from build123d import *

# Parameters (mm, degrees)
F1_DEPTH = 25


with BuildPart() as f1:
    # F0 (on Front) → F1 (new body)
    with BuildSketch(Plane.XZ):
        Polygon((42.157266, 36.458336), (0, 36.458336), (0, 32.877419), (39.633732, 32.877419), (39.633732, 12.629625), (35.397731, 12.629625), (35.397731, 8.376406), (39.750192, 8.376406), (39.750192, 6.429029), (39.750192, 6.314471), (49.760994, 6.314471), (49.760994, 8.376406), (49.683991, 10.766225), (42.157266, 10.766225), (42.157266, 12.629625), (42.157266, 14.715909), align=None)
    extrude(amount=F1_DEPTH)

    # F0 (on Front) → F2 (revolve)
    with BuildSketch(Plane.XZ):
        Polygon((42.157266, 36.458336), (0, 36.458336), (0, 32.877419), (39.633732, 32.877419), (39.633732, 12.629625), (35.397731, 12.629625), (35.397731, 8.376406), (39.750192, 8.376406), (39.750192, 6.429029), (39.750192, 6.314471), (49.760994, 6.314471), (49.760994, 8.376406), (49.683991, 10.766225), (42.157266, 10.766225), (42.157266, 12.629625), (42.157266, 14.715909), align=None)
    revolve(axis=Axis((0, 0, 20.221634), (0, 0, -1)))


solid = f1.part
Input: part model. Units: mm. Frame: model coordinates. A direction names the side the tool comes from. Round coordinates to 2 decimals unless told otherwise and drop trailing zeros. Loops run counter-clockwise (first coordinate to the right, second up) from the corner with the lowest first, then second, coordinate; pieces in that order, holes last. Notation, with made-up numbers: (0, 75) -> (23, 75) arc R4 ccw to (23, 80) -> close; hole circle Ø9 at (16.25, 74.25). An arc over 180 degrees is marked (long way). Answer as a JSON object with one key per item and string values. Group by question number.
1) Reachability of faces 5 (the flat face through (38, -22, 32.877)), 6 (the cylindrical face through (-31.54, 24.19, 7.33)), 7 (the flat face through (40, -25, 24)), 8 (the flat face through (1, -1, 32.877)) from +Z, -Z, +X, -X, +Y, -Y: full face, straight path, thin tool, end or side. Return the list, or none.
2) Pin query (flat end, axial travel): pin 1 (24 mm diameter, centred on x = -12.5, y = -19.5, fed in from -Z); pin 2 (8.5 mm diameter, centred on y = -18.5, z = 19, fed in from -X); pin 3 (4 mm diameter, centred on y = 1.5, z = 28, fed in from +X); pin 4 (1 mm diameter, centred on x = -25, y = 30.5, fed in from -Z). Return the tip coordinate at first contact, or that it passes through.
3) Ray query, L1, parallel to Y at x = 0, z = 7.9; L2, parallel to Y at x = 0, z = 11. Return the intervals inside material, ascending.
4) Draft query along Z for faces 1 (the conical face through (-48.467, 10.985, 10.385)), 2 (the cylindrical face through (33.763, -10.633, 10.473)), 3 (the flat face through (-14.9, -32.5, 12.63)), 4 (the flat face through (36, 3, 8.376)). Return one class per face: +Z half, -Z half, draft (parallel to the pull), parting line (faces both ways), or undercut.
5) Section query B-B on z = 19.5. Output: boundary loops of the cut face in (x, y).
6) Section query A-A on x = 0. Output: boundary loops of the cut face in (y, z), plus the area to 3 significant figures.
Reply:
{
 "1": {"face 5": "-Y", "face 6": "-Z", "face 7": "+Z, +X, -Y", "face 8": "none"},
 "2": {"pin 1": "stops at z = 32.88", "pin 2": "stops at x = -39.68", "pin 3": "stops at x = 42.16", "pin 4": "stops at z = 6.31"},
 "3": {"L1": "y = -49.76 to -39.75, 39.75 to 49.76", "L2": "y = -42.16 to -35.4, 35.4 to 42.16"},
 "4": {"face 1": "+Z half", "face 2": "draft", "face 3": "undercut", "face 4": "-Z half"},
 "5": {"outline": "(39.63, -25) -> (42.16, -25) -> (42.16, 0) arc R42.16 ccw (long way) to (39.63, -14.37) -> close; hole circle Ø79.27 at (0, 0)"},
 "6": {"outline": "(-49.76, 6.31) -> (-39.75, 6.31) -> (-39.75, 8.38) -> (-35.4, 8.38) -> (-35.4, 12.63) -> (-39.63, 12.63) -> (-39.63, 32.88) -> (39.63, 32.88) -> (39.63, 12.63) -> (35.4, 12.63) -> (35.4, 8.38) -> (39.75, 8.38) -> (39.75, 6.31) -> (49.76, 6.31) -> (49.76, 8.38) -> (49.68, 10.77) -> (42.16, 10.77) -> (42.16, 36.46) -> (-42.16, 36.46) -> (-42.16, 10.77) -> (-49.68, 10.77) -> (-49.76, 8.38) -> close", "area": "539 mm2"}
}
